```python
from build123d import *

# Parameters (mm, degrees)
CROQUIS1_W              = 45
CROQUIS1_H              = 45
CROQUIS1_W_2            = 35
CROQUIS1_H_2            = 35
SALIENTE_EXTRUIR1_DEPTH = 20
CORTAR_EXTRUIR1_DEPTH   = 46
CROQUIS6_W              = 35
CROQUIS6_H              = 25
CORTAR_EXTRUIR2_DEPTH   = 46
CROQUIS7_R              = 1
CORTAR_EXTRUIR3_DEPTH   = 46


with BuildPart() as part:
    # Croquis1 → Saliente-Extruir1 (new body, symmetric)
    with BuildSketch(Plane(origin=(0, 0, 0), x_dir=(1, 0, 0), z_dir=(0, 1, 0))):
        Rectangle(CROQUIS1_W, CROQUIS1_H)
        Rectangle(CROQUIS1_W_2, CROQUIS1_H_2, mode=Mode.SUBTRACT)
    extrude(amount=SALIENTE_EXTRUIR1_DEPTH, both=True)

    # Croquis3 → Cortar-Extruir1 (cut, through all)
    with BuildSketch(Plane(origin=(22.5, 0, 0), x_dir=(0, 0, -1), z_dir=(1, 0, 0))):
        Polygon((-22.5, -20), (22.5, -20), (22.5, 0.983844617), align=None)
    extrude(amount=-CORTAR_EXTRUIR1_DEPTH, mode=Mode.SUBTRACT)

    # Croquis6 → Cortar-Extruir2 (cut, through all)
    with BuildSketch(Plane.XY.offset(22.5)):
        with Locations((0, -7.5)):
            Rectangle(CROQUIS6_W, CROQUIS6_H)
    extrude(amount=-CORTAR_EXTRUIR2_DEPTH, mode=Mode.SUBTRACT)

    # Croquis7 → Cortar-Extruir3 (cut, through all)
    with BuildSketch(Plane(origin=(22.5, 0, 0), x_dir=(0, 0, -1), z_dir=(1, 0, 0))):
        with Locations((-20.307584971, -3)):
            Circle(CROQUIS7_R)
    extrude(amount=-CORTAR_EXTRUIR3_DEPTH, mode=Mode.SUBTRACT)


solid = part.part
```
Build history of the part. All positions in model axes, mm. A direction names the side the tool comes from. Give positions to 0.01 mm unless a question says otherwise; leave off trailing zeros. Order: outer loops, then holes, each group sorted by start corner. A loop starts at its lowest first (then second) coordinate and runs counter-clockwise, first axis right, second up. Notation, with made-up numbers: M 55,57.5 L 71,57.5 A34 cw 71,88.5 Z; hole C 82.25,73.5 d11. An arc over 180 degrees is marked long. Write item = value, one per line. Start each with the question number.
(1) Which spindle directions (+Z, -Z, +X, -X, +Y, -Y) get a long thin tool onto all of the face, cutting with end or side? Do faces 1 (the flat face through (0, 13, -22.5)), 2 (the flat face through (0, 9, 22.5)), 3 (the flat face through (-17.5, 4, 5)), 4 (the flat face through (0, 13, 17.5)), 5 (the flat face through (0, 5, 20)). Say none if no direction does.
(2) Slice it at D-D on y = -3. Write the cut outline in (x, z), plus the area to 3 significant figures.
(3) Pin check, flat tip, straight feed: pin 1 Ø1.5 at (x, z) = (-4, -21) entering from -Y. Stop position of the tip, or through.
(4) Slice it at C-C on x = -2.5. Write the cut outline in (y, z).
(5) Two-plate mould, pull along Z, no slides. Class faces 6 (the flat face through (17.5, 4, 5)), 7 (the flat face through (-19.965, -9.361, -0.315)), 8 (the flat face through (-22.5, 5, 0)), 9 (the cylindrical face through (-19.965, -2.956, 21.307)): released by +Z, released by -Z, zero draft, split by the parting line, or undercut.
(6) Slice it at A-A on y = 8.5. Write the cut outline in (x, z), plus the area to 3 significant figures.
(7) Probe L1, parallel to X at y = -2, z = 15; L2, parallel to Y at x = -15, z = -18. List the from-to ranges inside material, lowest first. Write a range as [from, to].
(8) Slice it at B-B on z = -10. Write the cut outline in (x, y) (3 decimals).
Responses:
q1.face_1 = -Z, +X, -X, +Y, -Y
q1.face_2 = +Z, +X, -X, +Y, -Y
q1.face_3 = -Y
q1.face_4 = +Y, -Y
q1.face_5 = +Z, -Z, -Y
q2.outline = M -22.5,-13.96 L -17.5,-13.96 L -17.5,19.31 L -22.5,19.31 Z; M -22.5,21.31 L -17.5,21.31 L -17.5,22.5 L -22.5,22.5 Z; M 17.5,-13.96 L 22.5,-13.96 L 22.5,19.31 L 17.5,19.31 Z; M 17.5,21.31 L 22.5,21.31 L 22.5,22.5 L 17.5,22.5 Z
q2.area = 345 mm2
q3.pin_1 = 5
q4.outline = M 5,-22.5 L 20,-22.5 L 20,-17.5 L 5,-17.5 Z; M 5,17.5 L 20,17.5 L 20,22.5 L 5,22.5 Z
q5.face_6 = undercut
q5.face_7 = released by -Z
q5.face_8 = zero draft
q5.face_9 = undercut
q6.outline = M -22.5,-22.5 L 22.5,-22.5 L 22.5,22.5 L -22.5,22.5 Z; hole M -17.5,-17.5 L 17.5,-17.5 L 17.5,17.5 L -17.5,17.5 Z
q6.area = 800 mm2
q7.L1 = [-22.5, -17.5], [17.5, 22.5]
q7.L2 = [5, 20]
q8.outline = M -22.5,-4.845 L -17.5,-4.845 L -17.5,20 L -22.5,20 Z; M 17.5,-4.845 L 22.5,-4.845 L 22.5,20 L 17.5,20 Z
